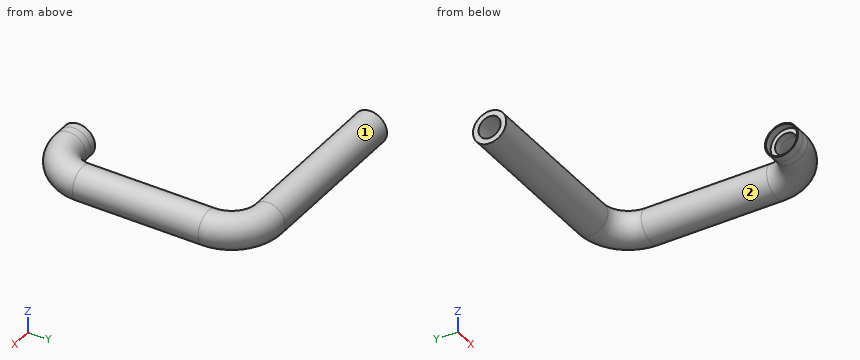
from build123d import *

# Parameters (mm, degrees)
SWEEP_THIN1_PROFILE_R    = 22.5
SWEEP_THIN1_PROFILE_R_2  = 15
BOSS_EXTRUDE1_DEPTH      = 10
BOSS_EXTRUDE1_DEPTH_BACK = 10
SKETCH6_R                = 22.5
SKETCH6_R_2              = 21


with BuildPart() as part:
    # Sweep-Thin1: sweep along a path in Sketch1
    with BuildLine(Plane.XY) as sweep_thin1_path:
        Line((0, 0), (220, 0))
        ThreePointArc((220, 0), (255.355339059, -14.644660941), (270, -50))
        Line((270, -50), (270, -220))
        ThreePointArc((270, -220), (255.355339059, -255.355339059), (220, -270))
        Line((220, -270), (210, -270))
    # Sweep-Thin1 profile (on start of the path) → Sweep-Thin1 (sweep)
    with BuildSketch(Plane(origin=(0, 0, 0), x_dir=(0, 0, 1), z_dir=(1, 0, 0))):
        Circle(SWEEP_THIN1_PROFILE_R)
        Circle(SWEEP_THIN1_PROFILE_R_2, mode=Mode.SUBTRACT)
    sweep(path=sweep_thin1_path.line)

    # Sketch6 → Boss-Extrude1 (add, two sides: drawn at the far end of the back side and taken through both)
    with BuildSketch(Plane.ZY.offset(-210).offset(-BOSS_EXTRUDE1_DEPTH_BACK)):
        with Locations((0, -270)):
            Circle(SKETCH6_R)
        with Locations((0, -270)):
            Circle(SKETCH6_R_2, mode=Mode.SUBTRACT)
    extrude(amount=BOSS_EXTRUDE1_DEPTH + BOSS_EXTRUDE1_DEPTH_BACK)


solid = part.part
Geometry check sheet. Reference: the model listing, model coordinates, mm. Face numbers are marked on the shaded views. A direction names the side the tool comes from. Round coordinates to 2 decimals unless told otherwise and drop trailing zeros. Write each loop counter-clockwise with the first axis right and the second up, starting at its lowest first coordinate (ties: lowest second). Pieces come first, ordered by that corner, then holes. Notation, with made-up numbers: (54, 41.5) -> (65, 41.5) arc R27 ccw to (65, 79.5) -> close; hole circle Ø4 at (87, 14). An arc over 180 degrees is marked (long way). One line per item, written item: value. Start each with the question number.
(1) Cross-section at B-B, the plane y = -90. Record the cut outline in (x, z), and give its area (3 significant figures).
(2) Scan lines: line 1 (Y direction, x = 204, z = 0); line 2 (Y direction, x = 140, z = 0); line 3 (X direction, y = -97.5, z = 0). Record each from-to range of solid material in increasing order. Write a range as [from, to].
(3) Cross-section at A-A, the plane z = 0. Record the cut outline in (x, y), and give its area (3 significant figures).
(4) Access from +Z, -Z, +X, -X, +Y, -Y to the whole of each face (thin tool, end or side, straight path). Record for the marked faces 1 and 2.
(5) Cross-section at D-D, the plane x = 236. Give the number of separate pieces and of enclosed holes in the cut face, and give its area (3 significant figures).
(6) Cross-section at C-C, the plane x = 82. Record the cut outline in (y, z), and give its area (3 significant figures).
(7) Go/stop test with flat-tipped pins: pin 1 Ø12 at (y, z) = (-133.5, -17) entering from +X; pin 2 Ø2 at (y, z) = (-63, -4) entering from +X; pin 3 Ø5 at (x, z) = (92.5, -13.5) entering from +Y. Record where each tip stops, or that it passes through.
Answer:
1. outline: circle Ø45 at (270, 0); hole circle Ø30 at (270, 0)
1. area: 884 mm²
2. line 1: [-292.5, -291], [-249, -247.5], [-22.5, -15], [15, 22.5]
2. line 2: [-22.5, -15], [15, 22.5]
2. line 3: [247.5, 255], [285, 292.5]
3. outline: (0, -22.5) -> (220, -22.5) arc R27.5 cw to (247.5, -50) -> (247.5, -220) arc R27.5 cw to (220, -247.5) -> (200, -247.5) -> (200, -249) -> (210, -249) -> (210, -255) -> (220, -255) arc R35 ccw to (255, -220) -> (255, -50) arc R35 ccw to (220, -15) -> (0, -15) -> close; (0, 15) -> (220, 15) arc R65 cw to (285, -50) -> (285, -220) arc R65 cw to (220, -285) -> (210, -285) -> (210, -291) -> (200, -291) -> (200, -292.5) -> (220, -292.5) arc R72.5 ccw to (292.5, -220) -> (292.5, -50) arc R72.5 ccw to (220, 22.5) -> (0, 22.5) -> close
3. area: 8,390 mm²
4. face 1: -X
4. face 2: none
5. separate pieces: 2
5. enclosed holes: 2
5. area: 1,900 mm²
6. outline: circle Ø45 at (0, 0); hole circle Ø30 at (0, 0)
6. area: 884 mm²
7. pin 1: x = 289.63
7. pin 2: x = 292.3
7. pin 3: y = 19.63
